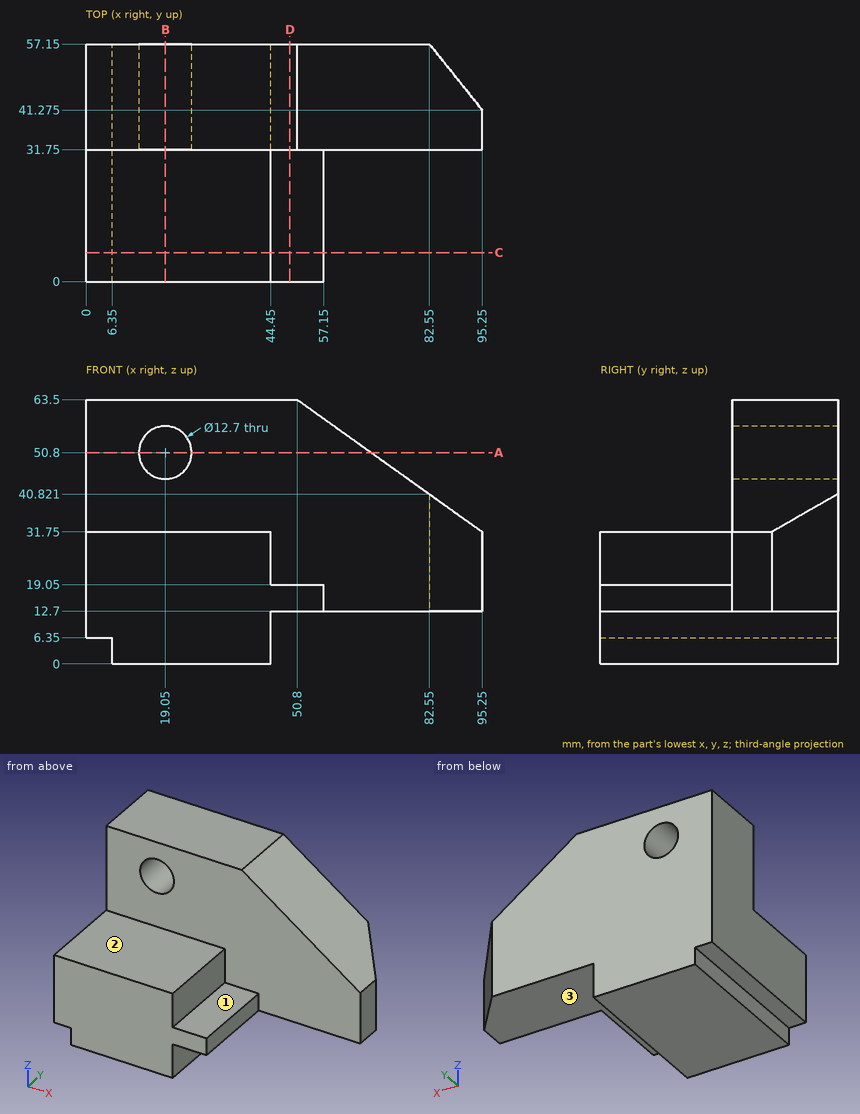
Could you check a few things on this drawing? It's one solid part, dimensions in mm from its lowest x, y, z. A direction names the side the tool comes from. Round coordinates to 2 decimals unless told otherwise and drop trailing zeros. Loops run counter-clockwise (first coordinate to the right, second up) from the corner with the lowest first, then second, coordinate; pieces in that order, holes last. Notation, with made-up numbers: M -8.75,-36 L 28.25,-36 A21 cw 28.25,-6 Z; hole C 79,67.5 d10. An arc over 180 degrees is marked long. Write item = value, one per line. Start each with the question number.
(1) Suppose I cut it at C-C on y = 7. Write out the boundary of the cut face in (x, z), plus the area to 3 significant figures.
(2) Suppose I cut it at A-A on z = 50.8. Write out the boundary of the cut face in (x, y), plus the area to 3 significant figures.
(3) I need wall thicknesses on line 1 along Z through (x, y) = (19.05, 39); line 2 along Z through (x, y) = (13.5, 32.5) (1 decimal); line 3 along Y through (x, z) = (63, 36.5). Which ranges of each line are inside material? Lowest first, please.
(4) Suppose I cut it at B-B on x = 19.05. Write out the boundary of the cut face in (y, z).
(5) I'm going to push flat-ended pins straight in: P1, Ø1.9, axis at y = 17.5, z = 2, coming from the -X side; P2, Ø4, axis at y = 39.5, z = 5, coming from the +X side; P3, Ø10, axis at x = 49.5, y = 12.5, coming from the +Z side; P4, Ø15, axis at x = 80, y = 19.5, coming from the -Z side. Where does each tip first touch, or does it pass through?
(6) Suppose I cut it at D-D on x = 49. Write out the boundary of the cut face in (y, z).
(7) Which directions (+Z, -Z, +X, -X, +Y, -Y) give clear straight access to the entire face, cutting with the end or side of a thin tool? Please do the marked faces 1, 2 and 3.
Answer block:
q1.outline = M 0,6.35 L 6.35,6.35 L 6.35,0 L 44.45,0 L 44.45,12.7 L 57.15,12.7 L 57.15,19.05 L 44.45,19.05 L 44.45,31.75 L 0,31.75 Z
q1.area = 1,450 mm²
q2.outline = M 0,31.75 L 12.7,31.75 L 12.7,57.15 L 0,57.15 Z; M 25.4,31.75 L 68.58,31.75 L 68.58,57.15 L 25.4,57.15 Z
q2.area = 1,420 mm²
q3.line_1 = 0 to 44.45, 57.15 to 63.5
q3.line_2 = 0 to 47.7, 53.9 to 63.5
q3.line_3 = 31.75 to 57.15
q4.outline = M 0,0 L 57.15,0 L 57.15,44.45 L 31.75,44.45 L 31.75,31.75 L 0,31.75 Z; M 31.75,57.15 L 57.15,57.15 L 57.15,63.5 L 31.75,63.5 Z
q5.P1 = 6.35
q5.P2 = 44.45
q5.P3 = 19.05
q5.P4 = through
q6.outline = M 0,12.7 L 57.15,12.7 L 57.15,63.5 L 31.75,63.5 L 31.75,19.05 L 0,19.05 Z
q7.face_1 = +Z, +X, -Y
q7.face_2 = +Z, +X, -X, -Y
q7.face_3 = -Z, +X, +Y, -Y
